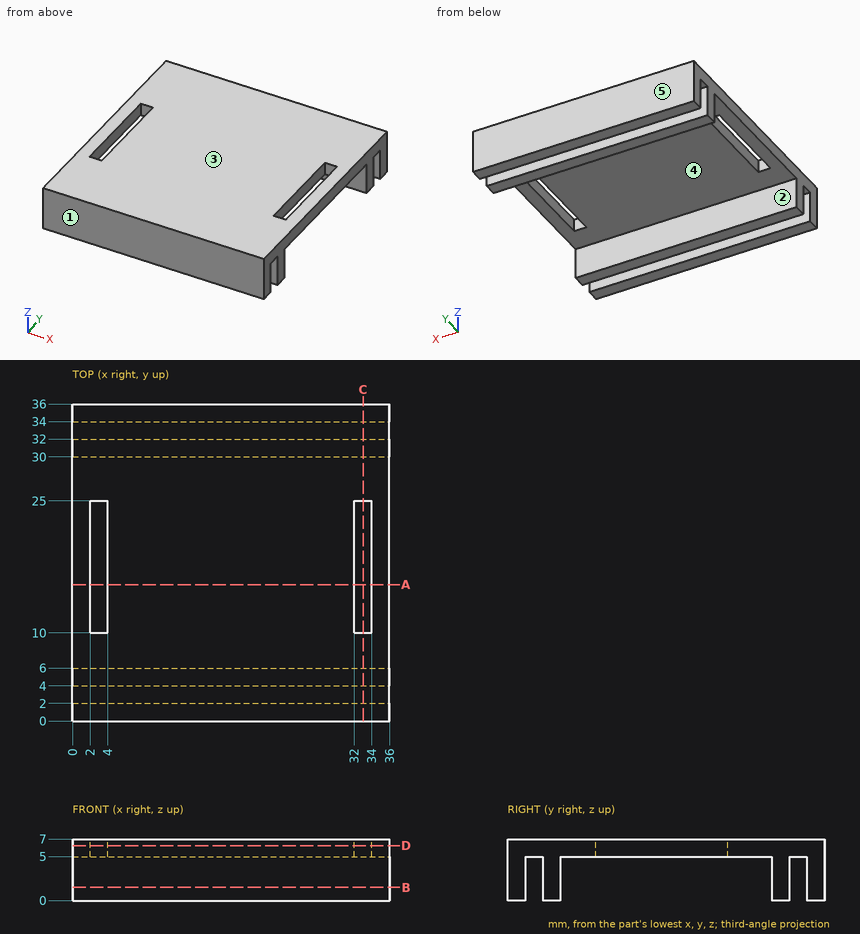
Design review of the part shown in the three views and the two pictorial views. Dimensions are in mm from the part's minimum x, y and z. A direction names the side the tool comes from. Round coordinates to 2 decimals unless told otherwise and drop trailing zeros. Write each loop counter-clockwise with the first axis right and the second up, starting at its lowest first coordinate (ties: lowest second). Pieces come first, ordered by that corner, then holes.
Item 1: Draft analysis for pull direction Y (two halves, no side actions). For the marked faces 3, 4 and 5, state which applies: released by +Y, released by -Y, zero draft, split by the parting line, or undercut.
Item 2: Consider section D-D on z = 6.25. Give the boundary of the cut face in (x, y).
Item 3: For the marked faces 1 and 2, list the 3-axis set-ups (+Z, -Z, +X, -X, +Y, -Y) from which the entire face can be reached by the end or side of a thin tool; tool diameter is ignored.
Item 4: Consider section B-B on z = 1.5. Give the boundary of the cut face in (x, y), and give its area (3 significant figures).
Item 5: Consider section C-C on x = 33. Give the boundary of the cut face in (y, z).
Item 6: Consider section A-A on y = 15.5. Give the boundary of the cut face in (x, z), and give its area (3 significant figures).
Item 7: Wall thickness on L1, parallel to Y at x = 24, z = 4.5; L2, parallel to X at y = 20.5, z = 5.5; L3, parallel to Y at x = 33, z = 6.5: over which ranges is each line inside the solid? List them lowest first.
Item 8: For pin 1 Ø1.5 at (x, z) = (9.5, 3.5) entering from -Y, flat-tipped, find the tip position at first contact; note if it passes through.
Check values:
1. face 3: zero draft
1. face 4: undercut
1. face 5: released by +Y
2. outline: (0, 0) - (36, 0) - (36, 36) - (0, 36) - close; hole (2, 10) - (4, 10) - (4, 25) - (2, 25) - close; hole (32, 10) - (34, 10) - (34, 25) - (32, 25) - close
3. face 1: +Z, -Z, +X, -X, -Y
3. face 2: -Z, +X, -X
4. outline: (0, 0) - (36, 0) - (36, 2) - (0, 2) - close; (0, 4) - (36, 4) - (36, 6) - (0, 6) - close; (0, 30) - (36, 30) - (36, 32) - (0, 32) - close; (0, 34) - (36, 34) - (36, 36) - (0, 36) - close
4. area: 288 mm2
5. outline: (0, 0) - (2, 0) - (2, 5) - (4, 5) - (4, 0) - (6, 0) - (6, 5) - (10, 5) - (10, 7) - (0, 7) - close; (25, 5) - (30, 5) - (30, 0) - (32, 0) - (32, 5) - (34, 5) - (34, 0) - (36, 0) - (36, 7) - (25, 7) - close
6. outline: (0, 5) - (2, 5) - (2, 7) - (0, 7) - close; (4, 5) - (32, 5) - (32, 7) - (4, 7) - close; (34, 5) - (36, 5) - (36, 7) - (34, 7) - close
6. area: 64.0 mm2
7. L1: y = 0 to 2, 4 to 6, 30 to 32, 34 to 36
7. L2: x = 0 to 2, 4 to 32, 34 to 36
7. L3: y = 0 to 10, 25 to 36
8. pin 1: stops at y = 0
